```python
from build123d import *

# Parameters (mm, degrees)
PAD_DEPTH = 5
FILLET_R  = 1


with BuildPart() as part:
    # Sketch → Pad (new body)
    with BuildSketch(Plane.XY):
        Polygon((0, 0), (7.5, 0), (7.5, 5), (5, 5), (5, 15), (128.5, 15), (128.5, 5), (126, 5), (126, 0), (133.5, 0), (133.5, 25), (118.5, 25), (118.5, 75), (116, 84.330127), (113.5, 75), (113.5, 25), (85.666667, 25), (85.666667, 75), (83.166667, 84.330127), (80.666667, 75), (80.666667, 25), (52.833333, 25), (52.833333, 75), (50.333333, 84.330127), (47.833333, 75), (47.833333, 25), (20, 25), (20, 75), (17.5, 84.330127), (15, 75), (15, 25), (0, 25), align=None)
    extrude(amount=PAD_DEPTH)

    # Fillet
    fillet_edges = [part.edges().sort_by_distance(p)[0] for p in [
        (0, 12.5, 5),
        (0, 12.5, 0),
        (3.75, 0, 5),
        (3.75, 0, 0),
        (7.5, 25, 5),
        (33.916667, 25, 5),
        (66.75, 25, 5),
        (99.583333, 25, 5),
        (126, 25, 5),
        (133.5, 12.5, 5),
        (129.75, 0, 5),
        (133.5, 0, 2.5),
        (129.75, 0, 0),
        (0, 0, 2.5),
        (7.5, 25, 0),
        (33.916667, 25, 0),
        (66.75, 25, 0),
        (99.583333, 25, 0),
        (126, 25, 0),
        (133.5, 25, 2.5),
        (133.5, 12.5, 0),
        (0, 25, 2.5),
        (128.5, 10, 0),
        (128.5, 10, 5),
        (5, 10, 0),
        (5, 10, 5),
    ]]
    fillet(fillet_edges, radius=FILLET_R)


solid = part.part
```
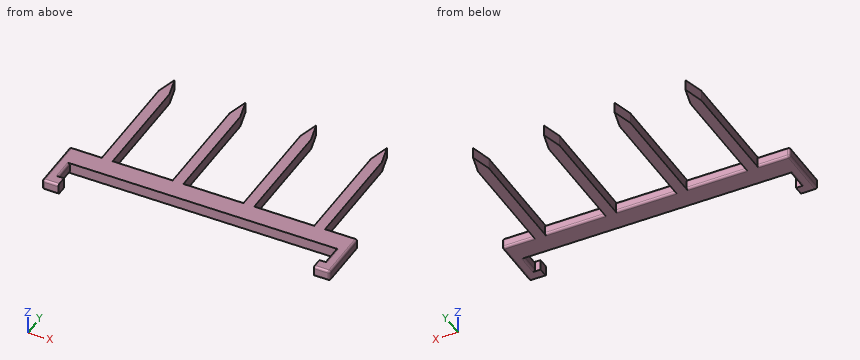
Part model, mm, in its own coordinate system. Coordinates: 2 decimals unless noted, no trailing zeros. Order: outer loops, then holes, each group sorted by start corner. A loop starts at its lowest first (then second) coordinate and runs counter-clockwise, first axis right, second up. Notation, with made-up numbers: (28.25, -39) - (33.25, -39) arc R19 ccw to (33.25, -14) - close; hole circle Ø8 at (22.5, -19). An arc over 180 degrees is marked (long way). Return JSON: item names as keys, results as strings. Group by question number.
Item 1: Cut at C-C (x = 99). List the corners of the cut face in (y, z).
Item 2: Drill centre lines: probe 1 along X at (y, z) = (39, 4.5); probe 2 along Y at (x, z) = (6.5, 3.7); probe 3 along X at (y, z) = (9.5, 2.8). Where is each one in solid material? Low to high. Write a range as from..to.
Item 3: Cut at B-B (y = 45). List the corners of the cut face in (x, z), plus the area to 3 significant figures.
Item 4: Pin check, flat tips, straight feed: pin 1 (1.5 mm diameter, centred on y = 46.5, z = 3.5, fed in from -X); pin 2 (0.9 mm diameter, centred on x = 66.5, z = 2, fed in from +Y); pin 3 (1.5 mm diameter, centred on y = 31, z = 1, fed in from +X). Stop position of each tip, or through.
Item 5: Cut at A-A (y = 8). List the corners of the cut face in (x, z), plus the area to 3 significant figures.
Check values:
{
 "1": {"outline": "(15, 0) - (24, 0) arc R1 ccw to (25, 1) - (25, 4) arc R1 ccw to (24, 5) - (15, 5) - close"},
 "2": {"probe 1": "x = 15..20, 47.83..52.83, 80.67..85.67, 113.5..118.5", "probe 2": "y = 0..5, 15..25", "probe 3": "x = 0..5, 128.5..133.5"},
 "3": {"outline": "(15, 0) - (20, 0) - (20, 5) - (15, 5) - close; (47.83, 0) - (52.83, 0) - (52.83, 5) - (47.83, 5) - close; (80.67, 0) - (85.67, 0) - (85.67, 5) - (80.67, 5) - close; (113.5, 0) - (118.5, 0) - (118.5, 5) - (113.5, 5) - close", "area": "100 mm2"},
 "4": {"pin 1": "stops at x = 15", "pin 2": "stops at y = 25", "pin 3": "stops at x = 118.5"},
 "5": {"outline": "(0, 1) arc R1 ccw to (1, 0) - (4, 0) arc R1 ccw to (5, 1) - (5, 4) arc R1 ccw to (4, 5) - (1, 5) arc R1 ccw to (0, 4) - close; (128.5, 1) arc R1 ccw to (129.5, 0) - (132.5, 0) arc R1 ccw to (133.5, 1) - (133.5, 4) arc R1 ccw to (132.5, 5) - (129.5, 5) arc R1 ccw to (128.5, 4) - close", "area": "48.3 mm2"}
}
